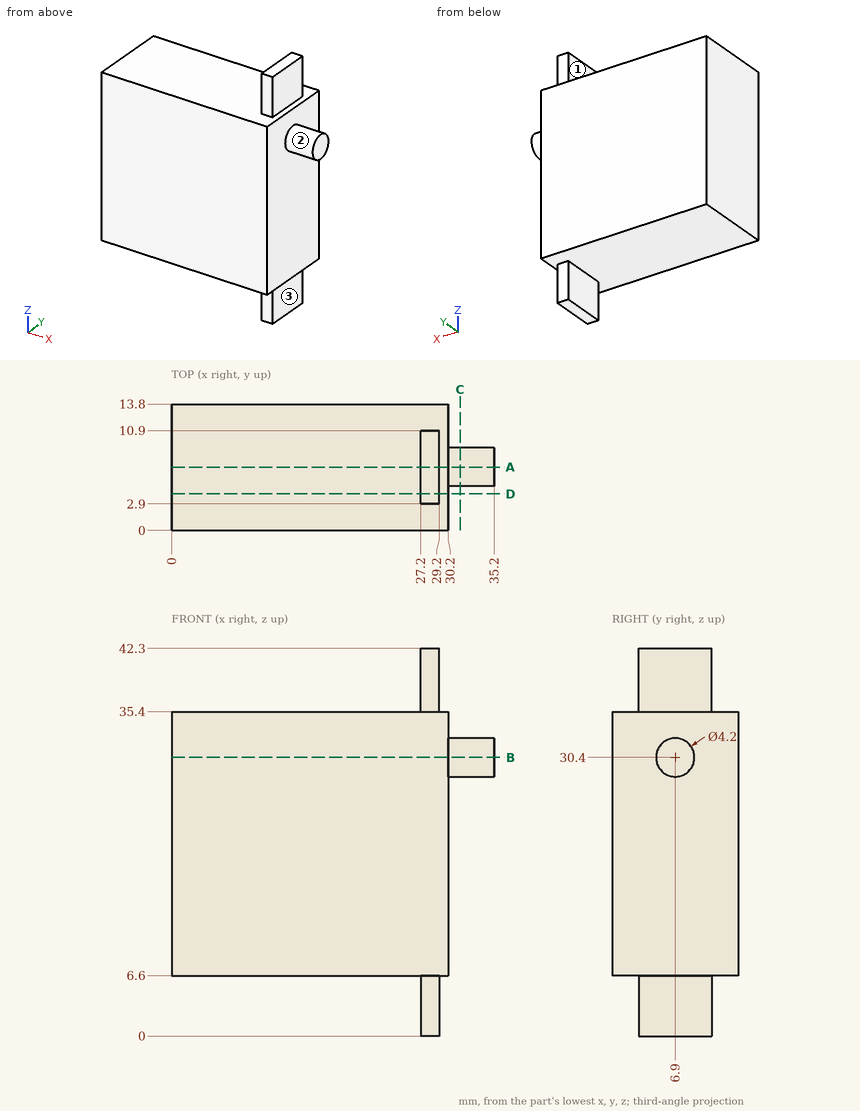
Could you check a few things on this drawing? It's one solid part, dimensions in mm from its lowest x, y, z. A direction names the side the tool comes from. Give positions to 0.01 mm unless a question says otherwise; leave off trailing zeros. Loops run counter-clockwise (first coordinate to the right, second up) from the corner with the lowest first, then second, coordinate; pieces in that order, holes last. Notation, with made-up numbers: (30.25, 83.5) -> (86.25, 83.5) arc R11 ccw to (86.25, 96.5) -> close; hole circle Ø6 at (-10, 58.5). An arc over 180 degrees is marked (long way). Use one line per item in the form item = value. Start each with the question number.
1) Imagine slicing it at C-C (x = 31.5). Please give me the cut outline in (y, z).
2) Imagine slicing it at B-B (z = 30.4). Please give me the cut outline in (x, y).
3) Which directions (+Z, -Z, +X, -X, +Y, -Y) give clear straight access to the entire face, cutting with the end or side of a thin tool? Please do the marked faces 1, 2 and 3.
4) For P1, Ø3.5, axis at y = 7, z = 3.5, coming from the +X side; P2, Ø1.5, axis at y = 4.5, z = 27.5, coming from the -X side; P3, Ø1, axis at x = 28, z = 37.5, coming from the -Y side; P4, Ø4, axis at x = 18, y = 10, coming from the -Z side, each with a flat end and sliding along its axis, tell me the tip position at first contact or that it passes through.
5) Imagine slicing it at D-D (y = 4). Please give me the cut outline in (x, z), then the cut area to 3 significant figures.
6) Imagine slicing it at A-A (y = 6.9). Please give me the cut outline in (x, z).
7) Please list where these lines run through material, in increasing order: line 1 along Z through (x, y) = (30, 2.25); line 2 along X through (y, z) = (12.25, 12); line 3 along X through (y, z) = (3.25, 35.5).
Check values:
q1.outline = circle Ø4.2 at (6.9, 30.4)
q2.outline = (0, 0) -> (30.2, 0) -> (30.2, 4.8) -> (35.2, 4.8) -> (35.2, 9) -> (30.2, 9) -> (30.2, 13.8) -> (0, 13.8) -> close
q3.face_1 = +Z, -X, +Y, -Y
q3.face_2 = +X
q3.face_3 = -Z, +X, +Y, -Y
q4.P1 = 29.2
q4.P2 = 0
q4.P3 = 2.9
q4.P4 = 6.6
q5.outline = (0, 6.6) -> (27.2, 6.6) -> (27.2, 0) -> (29.2, 0) -> (29.2, 6.6) -> (30.2, 6.6) -> (30.2, 35.4) -> (29.2, 35.4) -> (29.2, 42.3) -> (27.2, 42.3) -> (27.2, 35.4) -> (0, 35.4) -> close
q5.area = 897 mm^2
q6.outline = (0, 6.6) -> (27.2, 6.6) -> (27.2, 0) -> (29.2, 0) -> (29.2, 6.6) -> (30.2, 6.6) -> (30.2, 28.3) -> (35.2, 28.3) -> (35.2, 32.5) -> (30.2, 32.5) -> (30.2, 35.4) -> (29.2, 35.4) -> (29.2, 42.3) -> (27.2, 42.3) -> (27.2, 35.4) -> (0, 35.4) -> close
q7.line_1 = 6.6 to 35.4
q7.line_2 = 0 to 30.2
q7.line_3 = 27.2 to 29.2
